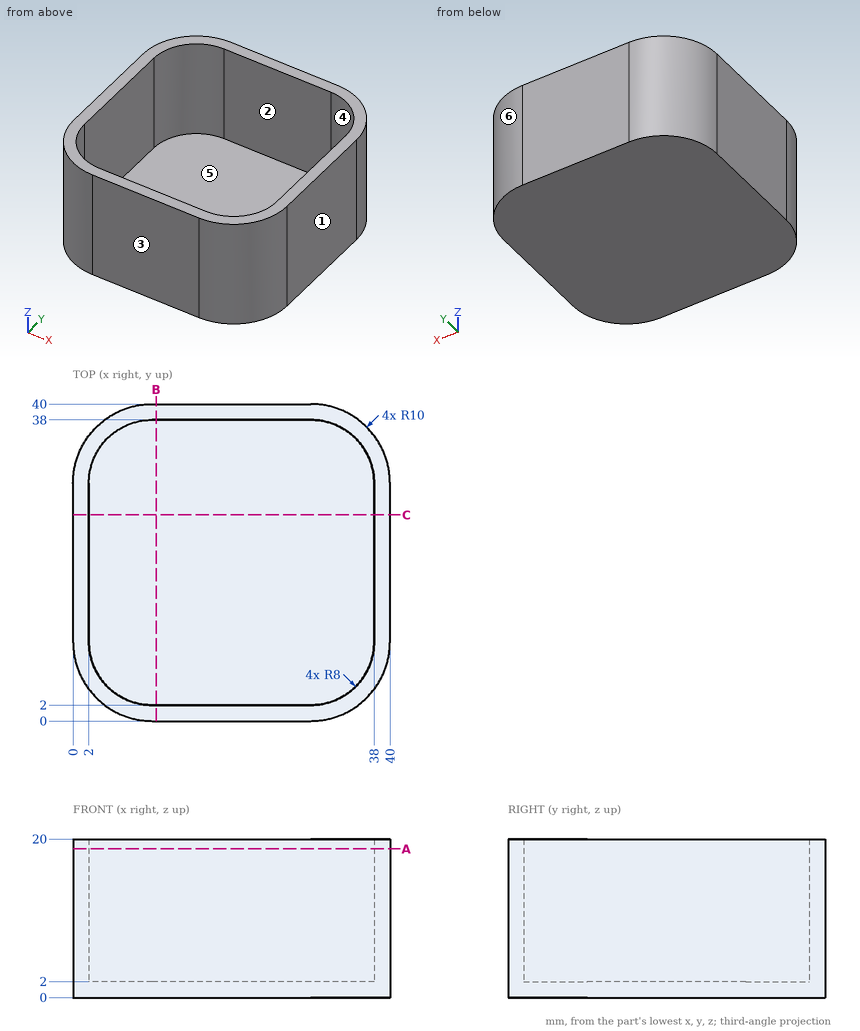
Could you check a few things on this drawing? It's one solid part, dimensions in mm from its lowest x, y, z. A direction names the side the tool comes from. Coordinates: 2 decimals unless noted, no trailing zeros. Loops run counter-clockwise (first coordinate to the right, second up) from the corner with the lowest first, then second, coordinate; pieces in that order, holes last.
1. We'd pull the mould along Y, two halves only. Please class the marked faces 1, 2, 3 and 4: released by +Y, released by -Y, zero draft, split by the parting line, or undercut.
2. For P1, Ø2, axis at x = 21, y = 26.5, coming from the -Z side; P2, Ø5, axis at y = 34.5, z = 2.5, coming from the -X side; P3, Ø8, axis at x = 8, y = 29, coming from the +Z side; P4, Ø1.5, axis at x = 7, z = 14.5, coming from the -Y side, each with a flat end and sliding along its axis, tell me the tip position at first contact or that it passes through.
3. I need wall thicknesses on L1, parallel to X at y = 15, z = 6.25; L2, parallel to Z at x = 26, y = 30. Which ranges of each line are inside material? Lowest first, please.
4. Imagine slicing it at A-A (z = 18.75). Please give me the cut outline in (x, y).
5. For the marked faces 5 and 6, which set-ups out of +Z, -Z, +X, -X, +Y, -Y let a thin tool reach every point of the face, with its end or its side?
6. Imagine slicing it at B-B (x = 10.5). Please give me the cut outline in (y, z), and give its area (3 significant figures).
Computed values:
1. face 1: zero draft
1. face 2: undercut
1. face 3: released by -Y
1. face 4: undercut
2. P1: stops at z = 0
2. P2: stops at x = 0.2
2. P3: stops at z = 2
2. P4: stops at y = 0.26
3. L1: x = 0 to 2, 38 to 40
3. L2: z = 0 to 2
4. outline: (0, 10) arc R10 ccw to (10, 0) - (30, 0) arc R10 ccw to (40, 10) - (40, 30) arc R10 ccw to (30, 40) - (10, 40) arc R10 ccw to (0, 30) - close; hole (2, 10) arc R8 ccw to (10, 2) - (30, 2) arc R8 ccw to (38, 10) - (38, 30) arc R8 ccw to (30, 38) - (10, 38) arc R8 ccw to (2, 30) - close
5. face 5: +Z
5. face 6: +Z, -Z, +X, +Y
6. outline: (0, 0) - (40, 0) - (40, 20) - (38, 20) - (38, 2) - (2, 2) - (2, 20) - (0, 20) - close
6. area: 152 mm2
